Can you work these out from the model? Positions are in its coordinate system, mm. Face numbers are marked on the shaded views. A direction names the side the tool comes from. Round coordinates to 2 decimals unless told otherwise and drop trailing zeros. Write each loop counter-clockwise with the first axis right and the second up, starting at its lowest first coordinate (ties: lowest second). Pieces come first, ordered by that corner, then holes. Notation, with made-up numbers: M 48,68 L 102,68 A6 ccw 102,79 Z; hole C -24.75,-7.5 d8. An arc over 180 degrees is marked long. Answer as a JSON object with one key per item and string values. Group by question number.
1) Suppose I cut it at A-A, the plane z = 0. Write out the boundary of the cut face in (x, y), and give its area (3 significant figures).
2) If we mould it in two halves opening along X, with no side actions, what happens to the marked faces 3, 4 and 5? For each: +X half, -X half, draft (parallel to the pull), parting line (faces both ways), or undercut.
3) Suppose I cut it at B-B, the plane y = 38. Write out the boundary of the cut face in (x, z), and give its area (3 significant figures).
4) I'm going to push flat-ended pins straight in: pin 1 Ø2.5 at (y, z) = (43.5, 0.5) entering from +X; pin 2 Ø4 at (y, z) = (16.5, -0.5) entering from +X; pin 3 Ø2.5 at (x, z) = (1, 0.5) entering from +Y; pin 4 Ø2 at (y, z) = (22.5, -2.5) entering from -X. Where does each tip first touch, or does it pass through?
5) Please list where these lines run through material, in increasing order: L1, parallel to Y at x = -1, z = 1.5; L2, parallel to Y at x = 1, z = -3.25; L3, parallel to X at y = 39, z = -1.5. Write a range as [from, to].
6) On a 3-axis mill with a long thin cutter (end or side, diameter ignored), from which of +Z, -Z, +X, -X, +Y, -Y can I reach the whole of each face in a straight line? I mean the marked faces 1 and 2. Say none if no direction works.
7) Suppose I cut it at D-D, the plane y = 27.5. Write out the boundary of the cut face in (x, z), and give its area (3 significant figures).
8) Suppose I cut it at C-C, the plane z = 4. Write out the boundary of the cut face in (x, y), and give its area (3 significant figures).
from build123d import *

# Parameters (mm, degrees)
ENL_V_MAT_EXTRU_1_DEPTH = 4


with BuildPart() as part:
    # Esquisse1 → Révolution1 (revolve)
    with BuildSketch(Plane.XY, mode=Mode.PRIVATE) as r_volution1_sk:
        Polygon((0, 0), (-2.45, 0), (-2.95, 0.5), (-2.95, 28), (-3, 28), (-3, 40), (-5, 40), (-5, 46), (0, 46), align=None)
    revolve(r_volution1_sk.sketch.rotate(Axis((0, 46, 0), (0, -1, 0)), 270), axis=Axis((0, 46, 0), (0, -1, 0)))

    # Esquisse2 → Enlèv. mat.-Extru.1 (cut)
    with BuildSketch(Plane(origin=(0, 46, 0), x_dir=(1, 0, 0), z_dir=(0, 1, 0))):
        Polygon((2.5, -1.443375673), (2.5, 1.443375673), (0, 2.886751346), (-2.5, 1.443375673), (-2.5, -1.443375673), (0, -2.886751346), align=None)
    extrude(amount=-ENL_V_MAT_EXTRU_1_DEPTH, mode=Mode.SUBTRACT)


solid = part.part
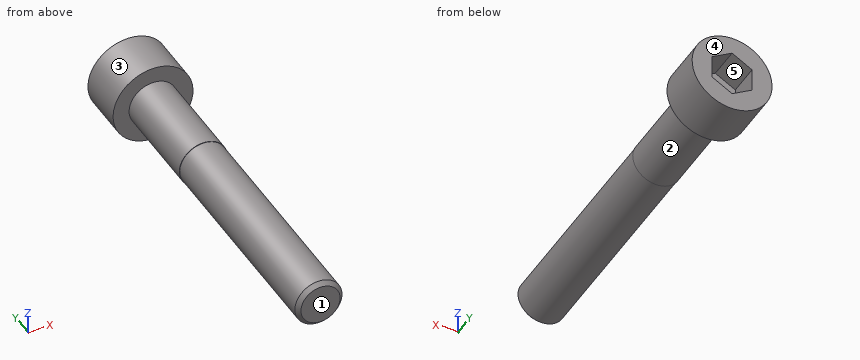
Results:
{
 "1": {"outline": "M -5,40 L -3,40 L -3,28 L -2.95,28 L -2.95,0.5 L -2.45,0 L 2.45,0 L 2.95,0.5 L 2.95,28 L 3,28 L 3,40 L 5,40 L 5,46 L 2.5,46 L 2.5,42 L -2.5,42 L -2.5,46 L -5,46 Z", "area": "277 mm^2"},
 "2": {"face 3": "parting line", "face 4": "draft", "face 5": "undercut"},
 "3": {"outline": "C 0,0 d6", "area": "28.3 mm^2"},
 "4": {"pin 1": "x = 5", "pin 2": "x = 2.95", "pin 3": "y = 42", "pin 4": "x = -2.54"},
 "5": {"L1": "[0, 42]", "L2": "[40, 46]", "L3": "[-2.6, 2.6]"},
 "6": {"face 1": "+Z, -Z, +X, -X, -Y", "face 2": "-Y"},
 "7": {"outline": "C 0,0 d5.9", "area": "27.3 mm^2"},
 "8": {"outline": "M -3,40 L 3,40 L 3,46 L -3,46 Z", "area": "36.0 mm^2"}
}
